Geometry: see drawing. Coordinates: mm, zero at the bounding-box minimum. Give positions to 0.01 mm unless a question says otherwise; leave off trailing zeros. Loops run counter-clockwise (first coordinate to the right, second up) from the corner with the lowest first, then second, coordinate; pieces in that order, holes last. Notation, with made-up numbers: (29.5, -27) -> (53.5, -27) arc R30 ccw to (53.5, 2) -> close; hole circle Ø1 at (51.25, 59). An arc over 180 degrees is marked (long way). One line per question, with ' | ' between items.
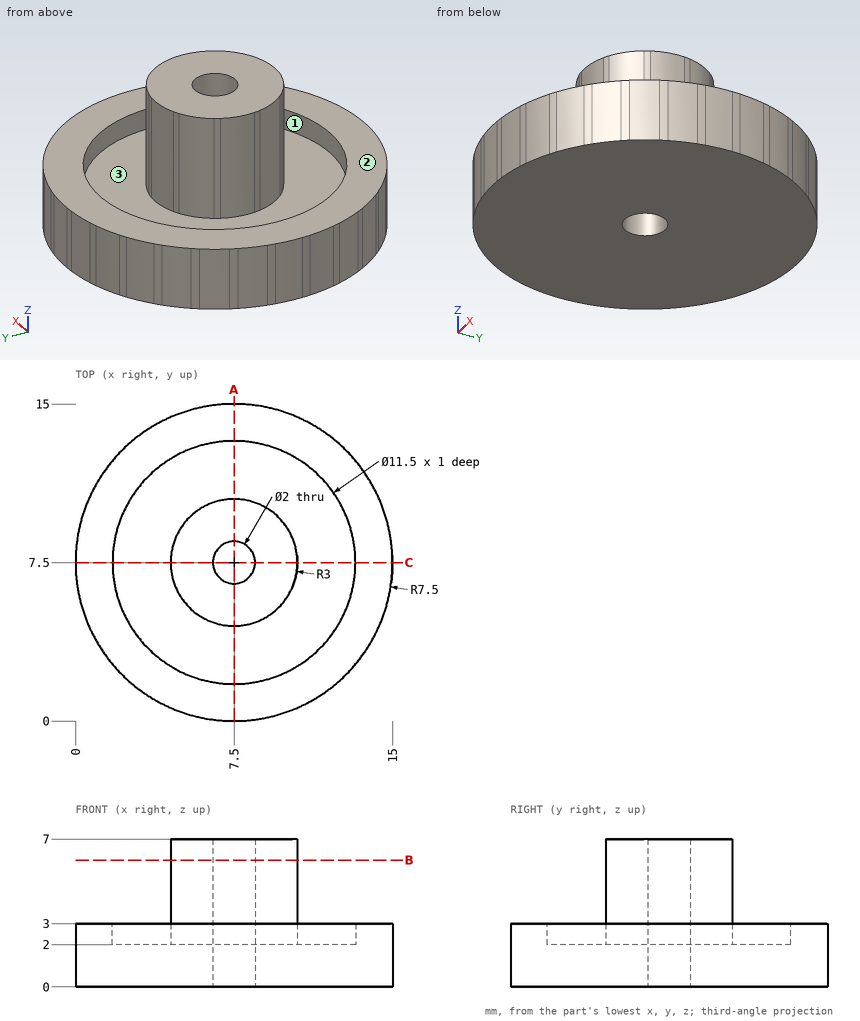
1. Ray query, line 1 along Y through (x, z) = (7.5, 2.65); line 2 along Y through (x, z) = (7.5, 3.5); line 3 along Y through (x, z) = (8.25, 1.75). Return the intervals inside material, ascending. Write a range as from..to.
Determined:
line 1: y = 0..1.75, 4.5..6.5, 8.5..10.5, 13.25..15 | line 2: y = 4.5..6.5, 8.5..10.5 | line 3: y = 0.04..6.84, 8.16..14.96
2. Pull-direction query (X, two-part tool) for the marked faces 1, 2 and 3; classes: pulls with the +X half, pulls with the -X half, needs draft (parallel to the pull), parting line crosses it, or undercut.
Determined:
face 1: undercut | face 2: needs draft | face 3: undercut
3. Pin query (flat end, axial travel): P1, Ø1.5, axis at x = 6.5, z = 3, coming from the +Y side; P2, Ø3, axis at x = 6.5, z = 5.5, coming from the -Y side. Return the tip coordinate at first contact, or that it passes through.
Determined:
P1: stops at y = 15 | P2: stops at y = 4.5
4. Section query A-A (x = 7.5). Output: boundary loops of the cut face in (y, z).
Determined:
outline: (0, 0) -> (6.5, 0) -> (6.5, 7) -> (4.5, 7) -> (4.5, 2) -> (1.75, 2) -> (1.75, 3) -> (0, 3) -> close; (8.5, 0) -> (15, 0) -> (15, 3) -> (13.25, 3) -> (13.25, 2) -> (10.5, 2) -> (10.5, 7) -> (8.5, 7) -> close
5. Section query B-B (z = 6). Output: boundary loops of the cut face in (x, y).
Determined:
outline: circle Ø6 at (7.5, 7.5); hole circle Ø2 at (7.5, 7.5)
